```python
from build123d import *

# Parameters (mm, degrees)
SKETCH1_W           = 90.3
SKETCH1_H           = 26
BOSS_EXTRUDE1_DEPTH = 20
SKETCH2_W           = 5
SKETCH2_H           = 20
CUT_EXTRUDE1_DEPTH  = 21
LPATTERN1_COUNT     = 2
LPATTERN1_PITCH     = 73.3
SKETCH3_R           = 6
CUT_EXTRUDE2_DEPTH  = 18
SKETCH4_W           = 19
SKETCH4_H           = 6
CUT_EXTRUDE3_DEPTH  = 22.5
SKETCH5_W           = 3
SKETCH5_H           = 8
BOSS_EXTRUDE2_DEPTH = 3
FILLET1_R           = 2


with BuildPart() as part:
    # Sketch1 → Boss-Extrude1 (new body)
    with BuildSketch(Plane(origin=(0, 0, 0), x_dir=(1, 0, 0), z_dir=(0, 1, 0))):
        with Locations((17.15729927, -0.427007299)):
            Rectangle(SKETCH1_W, SKETCH1_H)
    extrude(amount=-BOSS_EXTRUDE1_DEPTH)

    # Sketch2 → Cut-Extrude1 (cut, through all)
    with BuildSketch(Plane(origin=(0, 0, 0), x_dir=(1, 0, 0), z_dir=(0, 1, 0))):
        with Locations((53.80729927, -0.427007299)):
            Rectangle(SKETCH2_W, SKETCH2_H)
    cut_extrude1 = extrude(amount=-CUT_EXTRUDE1_DEPTH, mode=Mode.SUBTRACT)

    # LPattern1: Cut-Extrude1 ×2
    with Locations(*[(-i * LPATTERN1_PITCH, 0, 0) for i in range(1, LPATTERN1_COUNT)]):
        add(cut_extrude1, mode=Mode.SUBTRACT)

    # Sketch3 → Cut-Extrude2 (cut)
    with BuildSketch(Plane(origin=(0, 0, 0), x_dir=(1, 0, 0), z_dir=(0, 1, 0))):
        with Locations((38.30729927, 0)):
            Circle(SKETCH3_R)
        with Locations((-3.99270073, 0)):
            Circle(SKETCH3_R)
    extrude(amount=-CUT_EXTRUDE2_DEPTH, mode=Mode.SUBTRACT)

    # Sketch4 → Cut-Extrude3 (cut)
    with BuildSketch(Plane(origin=(0, 0, -12.572992701), x_dir=(-1, 0, 0), z_dir=(0, 0, -1))):
        with Locations((-38.80729927, -8.129091999)):
            Rectangle(SKETCH4_W, SKETCH4_H)
        with Locations((4.49270073, -8.129091999)):
            Rectangle(SKETCH4_W, SKETCH4_H)
    extrude(amount=-CUT_EXTRUDE3_DEPTH, mode=Mode.SUBTRACT)

    # Sketch5 → Boss-Extrude2 (add)
    with BuildSketch(Plane.XZ.offset(20)):
        with Locations((59.80729927, 0.427007299)):
            Rectangle(SKETCH5_W, SKETCH5_H)
        with Locations((-24.99270073, 0.427007299)):
            Rectangle(SKETCH5_W, SKETCH5_H)
    extrude(amount=BOSS_EXTRUDE2_DEPTH)

    # Fillet1
    fillet1_edges = [part.edges().sort_by_distance(p)[0] for p in [
        (62.30729927, 0, 0.427007299),
        (-27.99270073, 0, 0.427007299),
    ]]
    fillet(fillet1_edges, radius=FILLET1_R)


solid = part.part
```
The listing builds one solid part. Answer for the finished solid, in the listing's coordinates (mm). A direction names the side the tool comes from. Round coordinates to 2 decimals unless told otherwise and drop trailing zeros. Loops run counter-clockwise (first coordinate to the right, second up) from the corner with the lowest first, then second, coordinate; pieces in that order, holes last. Notation, with made-up numbers: (66, 85.5) - (109, 85.5) arc R27 ccw to (109, 124.5) - close; hole circle Ø10 at (24.5, 28.5). An arc over 180 degrees is marked (long way). Return JSON: item names as keys, results as strings. Group by question number.
1. The part is cut by section A-A on x = 52.5. Determine the outline of the cut face in (y, z), then the cut area to 3 significant figures.
2. The part is cut by section D-D on z = 0. State how many separate pieces and enclosed holes the cut face has, then the cut area to 3 significant figures.
3. Each of these flat-tipped pins is pushed along its axis until it touches: P1, Ø11, axis at x = -3.99, z = 0, coming from the +Y side; P2, Ø0.9, axis at y = -21, z = -1, coming from the -X side; P3, Ø4, axis at x = -12, z = 8.5, coming from the -Y side. Where does it stop, or does it pass through?
4. Consider probe 1 along X at (y, z) = (-8, -1); probe 2 along X at (y, z) = (-16, 0); probe 3 along X at (y, z) = (-18.5, 7). Determine where each line is inside the solid, lowest interval first.
5. Which of the six approach directions +Z, -Z, +X, -X, +Y, -Y give full straight-line access (tool end or side, diameter ignored) to faces 1 (the flat face through (54, -10, 10.427)), 2 (the flat face through (61.307, -21, 0)), 3 (the flat face through (-4.4, -5.129, -6.5)), 4 (the flat face through (-25, -21, -3.573)), 5 (the cylindrical face through (-5.29, -14.52, 5.86))?
6. The part is cut by section C-C on y = -6.5. Determine the outline of the cut face in (x, z).
7. The part is cut by section B-B on y = -13. Determine the outline of the cut face in (x, z).
8. The mould has two halves that part along X. Classify faces 6 (the flat face through (60, -21, 4.427)), 7 (the cylindrical face through (-27.42, -0.6, 0.25)), 8 (the flat face through (-20, -10, -9.573)): pulls with the +X half, pulls with the -X half, needs draft (parallel to the pull), parting line crosses it, or undercut.
Resolved:
{
 "1": {"outline": "(-20, -12.57) - (0, -12.57) - (0, -9.57) - (-20, -9.57) - close; (-20, 10.43) - (0, 10.43) - (0, 13.43) - (-20, 13.43) - close", "area": "120 mm²"},
 "2": {"separate pieces": "3", "enclosed holes": "0", "area": "1,110 mm²"},
 "3": {"P1": "stops at y = -18", "P2": "stops at x = -26.49", "P3": "stops at y = -20"},
 "4": {"probe 1": "x = -27.99 to -21.99, -16.99 to -13.99, 5.01 to 29.31, 48.31 to 51.31, 56.31 to 62.31", "probe 2": "x = -27.99 to -21.99, -16.99 to -9.99, 2.01 to 32.31, 44.31 to 51.31, 56.31 to 62.31", "probe 3": "x = -27.99 to -21.99, -16.99 to 51.31, 56.31 to 62.31"},
 "5": {"face 1": "+Y, -Y", "face 2": "+Z, -Z, +X, -Y", "face 3": "-Z", "face 4": "-Z, +X, -X, -Y", "face 5": "+Y"},
 "6": {"outline": "(-27.99, -12.57) - (-13.99, -12.57) - (-13.99, 9.93) - (5.01, 9.93) - (5.01, -12.57) - (29.31, -12.57) - (29.31, 9.93) - (48.31, 9.93) - (48.31, -12.57) - (62.31, -12.57) - (62.31, 13.43) - (-27.99, 13.43) - close; hole (-21.99, -9.57) - (-16.99, -9.57) - (-16.99, 10.43) - (-21.99, 10.43) - close; hole (51.31, -9.57) - (56.31, -9.57) - (56.31, 10.43) - (51.31, 10.43) - close"},
 "7": {"outline": "(-27.99, -12.57) - (62.31, -12.57) - (62.31, 13.43) - (-27.99, 13.43) - close; hole (-21.99, -9.57) - (-16.99, -9.57) - (-16.99, 10.43) - (-21.99, 10.43) - close; hole circle Ø12 at (-3.99, 0); hole circle Ø12 at (38.31, 0); hole (51.31, -9.57) - (56.31, -9.57) - (56.31, 10.43) - (51.31, 10.43) - close"},
 "8": {"face 6": "needs draft", "face 7": "pulls with the -X half", "face 8": "undercut"}
}
